Autodesk Inventor part; units mm, degrees
ref_plane "YZ Plane" through (0, 0, 0) normal (1, 0, 0) x (0, 1, 0)
ref_plane "XZ Plane" through (0, 0, 0) normal (0, 1, 0) x (-1, 0, 0)
ref_plane "XY Plane" through (0, 0, 0) normal (0, 0, 1) x (1, 0, 0)
ref_plane "Work Plane1" through (0, 0, 0) normal (0, 0, 1) x (1, 0, 0)
sketch "Sketch1" plane through (0, 0, 0) normal (0, 0, 1) x (1, 0, 0)
  line L0 (10, -5.5) -> (10, 39) construction
  line L1 (-10, 39) -> (10, 39) construction
  line L2 (-10, -5.5) -> (-10, 39) construction
  line L3 (-20.35, -5.5) -> (-10, -5.5)
  line L4 (-20.35, -19.6) -> (-20.35, -5.5)
  line L5 (20.35, -19.6) -> (-20.35, -19.6)
  line L6 (20.35, -19.6) -> (20.35, -5.5)
  line L7 (10, -5.5) -> (20.35, -5.5)
  line L8 (-20.35, -30.2) -> (-20.35, 45.6)
  line L9 (20.35, -30.2) -> (-20.35, -30.2)
  line L10 (-10, -5.5) -> (10, -5.5)
  line L11 (-20.35, -5.5) -> (-25.35, -5.5)
  line L12 (-25.35, -5.5) -> (-25.35, -35.2)
  line L13 (-25.35, -35.2) -> (-15.35, -35.2)
  line L14 (-15.35, -35.2) -> (-15.35, -30.2)
  line L15 (20.35, -19.6) -> (36.5729, -19.6)
  line L16 (36.5729, -19.6) -> (36.5729, 19)
  line L17 (36.5729, 19) -> (24.5729, 19)
  line L18 (24.5729, 19) -> (24.5729, -5.5)
  line L19 (24.5729, -5.5) -> (20.35, -5.5)
  line L20 (36.5729, 7) -> (24.5729, 7) construction
  line L21 (24.5729, 7) -> (24.5729, 19) construction
  line L22 (24.5729, 19) -> (36.5729, 19) construction
  line L23 (36.5729, 19) -> (36.5729, 7) construction
  point P0 (0, 0)
  dimension "d0" = 5
  dimension "d1" = 5
  dimension "d2" = 5
extrude "Extrusion1" add sketch "Sketch1" along normal blind 3
sketch "Sketch2" plane through (0, 0, 3) normal (0, 0, 1) x (1, 0, 0)
  line L0 (-15.35, -35.2) -> (-15.35, -30.2)
  line L1 (-15.35, -30.2) -> (-20.35, -30.2)
  line L2 (-20.35, -30.2) -> (-20.35, -19.6)
  line L3 (-20.35, -19.6) -> (36.5729, -19.6)
  line L4 (36.5729, -19.6) -> (36.5729, 19)
  line L5 (36.5729, 19) -> (24.5729, 19)
  line L6 (24.5729, 19) -> (24.5729, -5.5)
  line L7 (24.5729, -5.5) -> (-25.35, -5.5)
  line L8 (-25.35, -5.5) -> (-25.35, -35.2)
  line L9 (-25.35, -35.2) -> (-15.35, -35.2)
  point P0 (0, 0)
equation "\"d1\" = d0"
equation "\"d2\" = d0"
properties part number "Button Bracket 1" material "Wood (Oak)"
Can you work these out from the model? Positions are in its coordinate system, mm. A direction names the side the tool comes from. Give positions to 0.01 mm unless a question says otherwise; leave off trailing zeros. Write each loop counter-clockwise with the first axis right and the second up, starting at its lowest first coordinate (ties: lowest second). Pieces come first, ordered by that corner, then holes. Notation, with made-up numbers: (67.5, 81.25) -> (118.5, 81.25) arc R21 ccw to (118.5, 107.25) -> close; hole circle Ø9 at (64.5, -28). An arc over 180 degrees is marked (long way). One line per item, written item: value.
Q1. Imagine slicing it at B-B on y = 10. Please give me the cut outline in (x, z), and give its area (3 significant figures).
Results found:
outline: (24.57, 0) -> (36.57, 0) -> (36.57, 3) -> (24.57, 3) -> close
area: 36.0 mm^2
Q2. Please list where these lines run through material, in increasing order: line 1 (Y direction, x = -18, z = 1.75); line 2 (X direction, y = -1.5, z = 0.45); line 3 (Y direction, x = 22, z = 1.4). Write a range as [from, to].
Results found:
line 1: y = [-35.2, -30.2], [-19.6, -5.5]
line 2: x = [24.57, 36.57]
line 3: y = [-19.6, -5.5]
Q3. Which directions (+Z, -Z, +X, -X, +Y, -Y) give clear straight access to the entire face, cutting with the end or side of a thin tool? Please do faces 1 (the face through (-18, -30.2, 1)), 2 (the face through (-15.35, -33, 1)), 3 (the face through (24.573, 7, 1)), 4 (the face through (-20, -35.2, 1)), 5 (the face through (5, -8, 3)).
Results found:
face 1: +Z, -Z, +X
face 2: +Z, -Z, +X, -Y
face 3: +Z, -Z, -X, +Y
face 4: +Z, -Z, +X, -X, -Y
face 5: +Z, +X, -X, +Y, -Y
Q4. Imagine slicing it at A-A on z = 1.05. Please give me the cut outline in (x, y), and give its area (3 significant figures).
Results found:
outline: (-25.35, -35.2) -> (-15.35, -35.2) -> (-15.35, -30.2) -> (-20.35, -30.2) -> (-20.35, -19.6) -> (36.57, -19.6) -> (36.57, 19) -> (24.57, 19) -> (24.57, -5.5) -> (-25.35, -5.5) -> close
area: 1,270 mm^2
Q5. For P1, Ø0.9, axis at y = 10, z = 2, coming from the -X side; P2, Ø1, axis at x = 22, z = 1, coming from the -Y side; P3, Ø1.5, axis at y = -33.5, z = 1.5, coming from the +X side, each with a flat end and sliding along its axis, tell me the tip position at first contact or that it passes through.
Results found:
P1: stops at x = 24.57
P2: stops at y = -19.6
P3: stops at x = -15.35
Q6. Imagine slicing it at C-C on x = 27. Please give me the cut outline in (y, z), and give its area (3 significant figures).
Results found:
outline: (-19.6, 0) -> (19, 0) -> (19, 3) -> (-19.6, 3) -> close
area: 116 mm^2
